Verification items for the finished model (mm, model axes). A direction names the side the tool comes from. Round coordinates to 2 decimals unless told otherwise and drop trailing zeros. Order: outer loops, then holes, each group sorted by start corner. A loop starts at its lowest first (then second) coordinate and runs counter-clockwise, first axis right, second up. Notation, with made-up numbers: M 77.25,-28 L 99.25,-28 A23 cw 99.25,1 Z; hole C 69.25,61 d11. An arc over 180 degrees is marked long. Write item = value, one per line. Start each with the question number.
from build123d import *

# Parameters (mm, degrees)
SKETCH2_W               = 70
SKETCH2_H               = 45
BOSS_EXTRUDE1_DEPTH     = 1.6
SKETCH3_R               = 3.125
CUT_EXTRUDE1_DEPTH      = 1.6
SKETCH4_W               = 70
SKETCH4_H               = 45
SKETCH4_W_2             = 66.8
SKETCH4_H_2             = 41.8
BOSS_EXTRUDE2_DEPTH     = 28.15
BOSS_EXTRUDE3_START     = 16.5
SKETCH5_R               = 4.25
SKETCH5_R_2             = 3.125
BOSS_EXTRUDE3_DEPTH     = 16.5
BOSS_EXTRUDE4_START     = 2
SKETCH6_R               = 4.25
SKETCH6_R_2             = 1.75
BOSS_EXTRUDE4_DEPTH     = 2
CHAMFER1_SIZE           = 1.5
SKETCH7_R               = 7
CUT_EXTRUDE2_DEPTH      = 10
CUT_EXTRUDE3_DEPTH      = 28.15
CUT_EXTRUDE4_DEPTH      = 64.195114526
CUT_EXTRUDE4_DEPTH_BACK = 64.195114526
SKETCH9_R               = 2.8
SKETCH10_R              = 5
SKETCH10_R_2            = 2.8
BOSS_EXTRUDE5_DEPTH     = 2
CHAMFER2_SIZE           = 2
SKETCH11_W              = 2
SKETCH11_H              = 3
SKETCH11_H_2            = 10.952479139
BOSS_EXTRUDE6_DEPTH     = 10


# Some blends are built 0.0001 mm under size
with BuildPart() as part:
    # Sketch2 → Boss-Extrude1 (new body)
    with BuildSketch(Plane.XY):
        Rectangle(SKETCH2_W, SKETCH2_H)
    extrude(amount=BOSS_EXTRUDE1_DEPTH)

    # Sketch3 → Cut-Extrude1 (cut)
    with BuildSketch(Plane.XY.offset(1.6)):
        with Locations((-22.5, 13.5)):
            Circle(SKETCH3_R)
        with Locations((28.5, 13.5)):
            Circle(SKETCH3_R)
        with Locations((28.5, -13.5)):
            Circle(SKETCH3_R)
    extrude(amount=-CUT_EXTRUDE1_DEPTH, mode=Mode.SUBTRACT)

    # Sketch4 → Boss-Extrude2 (add)
    with BuildSketch(Plane.XY.offset(1.6)):
        Rectangle(SKETCH4_W, SKETCH4_H)
        Rectangle(SKETCH4_W_2, SKETCH4_H_2, mode=Mode.SUBTRACT)
    extrude(amount=BOSS_EXTRUDE2_DEPTH)

    # Sketch5 → Boss-Extrude3 (add)
    # profile 1 of 3: a face of its own
    with BuildSketch(Plane.XY.offset(1.6).offset(BOSS_EXTRUDE3_START)):
        with Locations((-22.5, 13.5)):
            Circle(SKETCH5_R)
        with Locations((-22.5, 13.5)):
            Circle(SKETCH5_R_2, mode=Mode.SUBTRACT)
    # profile 2 of 3: a face of its own
    with BuildSketch(Plane.XY.offset(1.6).offset(BOSS_EXTRUDE3_START)):
        with Locations((28.5, 13.5)):
            Circle(SKETCH5_R)
        with Locations((28.5, 13.5)):
            Circle(SKETCH5_R_2, mode=Mode.SUBTRACT)
    # profile 3 of 3: a face of its own
    with BuildSketch(Plane.XY.offset(1.6).offset(BOSS_EXTRUDE3_START)):
        with Locations((28.5, -13.5)):
            Circle(SKETCH5_R)
        with Locations((28.5, -13.5)):
            Circle(SKETCH5_R_2, mode=Mode.SUBTRACT)
    extrude(amount=-BOSS_EXTRUDE3_DEPTH)

    # Sketch6 → Boss-Extrude4 (add)
    # profile 1 of 3: a face of its own
    with BuildSketch(Plane.XY.offset(18.1).offset(BOSS_EXTRUDE4_START)):
        with Locations((28.5, -13.5)):
            Circle(SKETCH6_R)
        with Locations((28.5, -13.5)):
            Circle(SKETCH6_R_2, mode=Mode.SUBTRACT)
    # profile 2 of 3: a face of its own
    with BuildSketch(Plane.XY.offset(18.1).offset(BOSS_EXTRUDE4_START)):
        with Locations((28.5, 13.5)):
            Circle(SKETCH6_R)
        with Locations((28.5, 13.5)):
            Circle(SKETCH6_R_2, mode=Mode.SUBTRACT)
    # profile 3 of 3: a face of its own
    with BuildSketch(Plane.XY.offset(18.1).offset(BOSS_EXTRUDE4_START)):
        with Locations((-22.5, 13.5)):
            Circle(SKETCH6_R)
        with Locations((-22.5, 13.5)):
            Circle(SKETCH6_R_2, mode=Mode.SUBTRACT)
    extrude(amount=-BOSS_EXTRUDE4_DEPTH)

    # Chamfer1
    # the kernel refuses this chamfer: 1.5 mm, written as the material it takes off along each edge
    with BuildSketch(Plane(origin=(28.5, 13.5, 18.1), x_dir=(1, 0, 0), z_dir=(0, -1, 0))) as chamfer1_piece_1_section:
        Polygon((1.75, CHAMFER1_SIZE), (1.75 + CHAMFER1_SIZE, 0), (1.75, 0), align=None)
    chamfer1_piece_1 = revolve(axis=Axis((28.5, 13.5, 18.1), (0, 0, 1)), mode=Mode.PRIVATE)
    chamfer1_piece_1 = chamfer1_piece_1 & Plane(origin=(28.5, 13.5, 18.915495492), x_dir=(1, 0, 0), z_dir=(0, 0, 1)) * Cylinder(3.125, 13, mode=Mode.PRIVATE)
    add(chamfer1_piece_1, mode=Mode.SUBTRACT)
    with BuildSketch(Plane(origin=(28.5, -13.5, 18.1), x_dir=(1, 0, 0), z_dir=(0, -1, 0))) as chamfer1_piece_2_section:
        Polygon((1.75, CHAMFER1_SIZE), (1.75 + CHAMFER1_SIZE, 0), (1.75, 0), align=None)
    chamfer1_piece_2 = revolve(axis=Axis((28.5, -13.5, 18.1), (0, 0, 1)), mode=Mode.PRIVATE)
    chamfer1_piece_2 = chamfer1_piece_2 & Plane(origin=(28.5, -13.5, 18.915495492), x_dir=(1, 0, 0), z_dir=(0, 0, 1)) * Cylinder(3.125, 13, mode=Mode.PRIVATE)
    add(chamfer1_piece_2, mode=Mode.SUBTRACT)
    with BuildSketch(Plane(origin=(-22.5, 13.5, 18.1), x_dir=(1, 0, 0), z_dir=(0, -1, 0))) as chamfer1_piece_3_section:
        Polygon((1.75 + CHAMFER1_SIZE, 0), (1.75, CHAMFER1_SIZE), (1.75, 0), align=None)
    chamfer1_piece_3 = revolve(axis=Axis((-22.5, 13.5, 18.1), (0, 0, 1)), mode=Mode.PRIVATE)
    chamfer1_piece_3 = chamfer1_piece_3 & Plane(origin=(-22.5, 13.5, 18.915495492), x_dir=(1, 0, 0), z_dir=(0, 0, 1)) * Cylinder(3.125, 13, mode=Mode.PRIVATE)
    add(chamfer1_piece_3, mode=Mode.SUBTRACT)

    # Sketch7 → Cut-Extrude2 (cut)
    with BuildSketch(Plane(origin=(35, 0, 0), x_dir=(0, 0, -1), z_dir=(1, 0, 0))):
        with Locations((-29.75, 1.13)):
            Circle(SKETCH7_R)
    extrude(amount=-CUT_EXTRUDE2_DEPTH, mode=Mode.SUBTRACT)

    # Sketch8 → Cut-Extrude3 (cut)
    with BuildSketch(Plane.XY.offset(29.75)):
        Polygon((-35, -18.976239569), (-33.4, -19.9), (-33.4, 11.947520861), (-35, 11.023760431), align=None)
    extrude(amount=-CUT_EXTRUDE3_DEPTH, mode=Mode.SUBTRACT)

    # Sketch9 → Cut-Extrude4 (cut, two sides: drawn at the far end of the back side and taken through both)
    with BuildSketch(Plane.XZ.offset(-20.9).offset(-CUT_EXTRUDE4_DEPTH_BACK)):
        with Locations(Location((0, 15.675, 0), (0, 0, 270))):
            Circle(SKETCH9_R)
    extrude(amount=CUT_EXTRUDE4_DEPTH + CUT_EXTRUDE4_DEPTH_BACK, mode=Mode.SUBTRACT)

    # Sketch10 → Boss-Extrude5 (add)
    with BuildSketch(Plane.XZ.offset(-20.9)):
        with Locations(Location((0, 15.675, 0), (0, 0, 270))):
            Circle(SKETCH10_R)
        with Locations(Location((0, 15.675, 0), (0, 0, 270))):
            Circle(SKETCH10_R_2, mode=Mode.SUBTRACT)
    extrude(amount=BOSS_EXTRUDE5_DEPTH)

    # Chamfer2
    chamfer2_edges = [part.edges().sort_by_distance(p)[0] for p in [
        (0, 20.9, 20.675),
    ]]
    chamfer(chamfer2_edges, length=CHAMFER2_SIZE - 0.0001)  # a hair under: the kernel refuses the full size

    # Sketch11 → Boss-Extrude6 (add)
    with BuildSketch(Plane.XY.offset(1.6)):
        with Locations((-32.4, -19.4)):
            Rectangle(SKETCH11_W, SKETCH11_H)
        with Locations((-32.4, 15.423760431)):
            Rectangle(SKETCH11_W, SKETCH11_H_2)
    extrude(amount=BOSS_EXTRUDE6_DEPTH)


solid = part.part
1) Cross-section at A-A, the plane x = -22.5. Enter the section's corners in (y, z) (3 decimals), then the cut area to 3 significant figures.
2) Scan lines: probe 1 along Y at (x, z) = (28.5, 7.75) (3 decimals); probe 2 along X at (y, z) = (17, 13.25); probe 3 along Y at (x, z) = (28.5, 20.5). Record each from-to range of solid material in increasing order.
3) Cross-section at C-C, the plane x = 28.5. Give the number of separate pieces and of enclosed holes in the cut face, then the cut area to 3 significant figures.
4) Access from +Z, -Z, +X, -X, +Y, -Y to the whole of each face (thin tool, end or side, straight path). Record for faces 1 (the cylindrical face through (34.21, 0.98, 22.75)), 2 (the flat face through (0, -20.9, 19)), 3 (the flat face through (30.3, -14.4, 20.1)), 4 (the cylindrical face through (31.48, 14.44, 9.24)), 5 (the cylindrical face through (27.21, 14.68, 19.85)).
5) Cross-section at D-D, the plane z = 25.5. Enter the section's corners in (x, y).
6) Release check for a two-part mould opening along Y. For faces 6 (the conical face through (1.539, 19.025, 10.787)), 7 (the flat face through (0, 0, 0)) record: pulls with the +Y half, pulls with the -Y half, needs draft (parallel to the pull), parting line crosses it, or undercut.
7) Cross-section at B-B, the plane y = -13.5. Enter the section's corners in (x, z) (3 decimals), then the cut area to 3 significant figures.
8) Gauge pin test, flat ends, axial feed: P1, Ø0.6, axis at x = -33, y = 14.5, coming from the +Z side; P2, Ø5, axis at x = -6, y = 3.5, coming from the +Z side; P3, Ø5, axis at x = -22.5, y = 13.5, coming from the -Z side. Record the tip position at first contact, or that the pin passes through.
Geometry results:
q1.outline = M -22.5,0 L 10.375,0 L 10.375,18.225 L 11.75,19.6 L 11.75,20.1 L 9.25,20.1 L 9.25,1.6 L -20.9,1.6 L -20.9,29.75 L -22.5,29.75 Z; M 15.25,19.6 L 16.625,18.225 L 16.625,0 L 22.5,0 L 22.5,29.75 L 20.9,29.75 L 20.9,1.6 L 17.75,1.6 L 17.75,20.1 L 15.25,20.1 Z
q1.area = 197 mm^2
q2.probe_1 = -22.5 to -20.9, -17.75 to -16.625, -10.375 to -9.25, 9.25 to 10.375, 16.625 to 17.75, 20.9 to 22.5
q2.probe_2 = -35 to -33.4, -24.91 to -20.09, 26.09 to 30.91, 33.4 to 35
q2.probe_3 = -22.5 to -20.9, 20.9 to 22.5
q3.separate_pieces = 3
q3.enclosed_holes = 0
q3.area = 232 mm^2
q4.face_1 = +Z, +X, -X
q4.face_2 = +Z
q4.face_3 = +Z, -X
q4.face_4 = -Z
q4.face_5 = +Z, -Z
q5.outline = M -35,-22.5 L 35,-22.5 L 35,-4.43 L 33.4,-4.43 L 33.4,-20.9 L -33.4,-20.9 L -33.4,-19.9 L -35,-18.98 Z; M -35,11.02 L -33.4,11.95 L -33.4,20.9 L 33.4,20.9 L 33.4,6.69 L 35,6.69 L 35,22.5 L -35,22.5 Z
q6.face_6 = undercut
q6.face_7 = needs draft
q7.outline = M -35,0 L 25.375,0 L 25.375,18.225 L 26.75,19.6 L 26.75,20.1 L 24.25,20.1 L 24.25,1.6 L -35,1.6 Z; M 30.25,19.6 L 31.625,18.225 L 31.625,0 L 35,0 L 35,29.75 L 33.4,29.75 L 33.4,1.6 L 32.75,1.6 L 32.75,20.1 L 30.25,20.1 Z
q7.area = 192 mm^2
q8.P1 = 11.6
q8.P2 = 1.6
q8.P3 = 18.85
